from build123d import *

# Parameters (mm, degrees)
F0_R     = 2.5
F3_DEPTH = 24
F1_R     = 11
F4_DEPTH = 2
F5_DEPTH = 47
F7_D     = 4


with BuildPart() as f3:
    # F0 (on Front) → F3 (new body)
    with BuildSketch(Plane.XZ):
        Circle(F0_R)
    extrude(amount=F3_DEPTH)

    # F1 (on Front) → F4 (join)
    with BuildSketch(Plane.XZ):
        Circle(F1_R)
    extrude(amount=F4_DEPTH)

    # F2 (on Front) → F5 (join)
    with BuildSketch(Plane.XZ):
        Polygon((21, 16.5), (16.5, 21), (-16.5, 21), (-21, 16.5), (-21, -16.5), (-16.5, -21), (16.5, -21), (21, -16.5), align=None)
    extrude(amount=-F5_DEPTH)

    # F7 (through all)
    with Locations(Plane.XZ):
        with Locations((-15.5, 15.5), (15.5, 15.5), (15.5, -15.5), (-15.5, -15.5)):
            Hole(F7_D / 2)


solid = f3.part
For this review, take the finished solid that the model builds, in its own axes (mm). A direction names the side the tool comes from. Round coordinates to 2 decimals unless told otherwise and drop trailing zeros. Write each loop counter-clockwise with the first axis right and the second up, starting at its lowest first coordinate (ties: lowest second). Pieces come first, ordered by that corner, then holes. Notation, with made-up numbers: (38, -32) -> (43, -32) arc R28 ccw to (43, 4) -> close; hole circle Ø9 at (73, 39). An arc over 180 degrees is marked (long way). Put each result on its own line as item: value.
Q1. To check wall thickness, follow L1, parallel to Z at x = 15.5, y = 15; L2, parallel to Z at x = 15, y = 32. State the ranges of each line that lie inside material, in increasing order. Write a range as [from, to].
Determined:
L1: z = [-21, -17.5], [-13.5, 13.5], [17.5, 21]
L2: z = [-21, -17.44], [-13.56, 13.56], [17.44, 21]
Q2. Consider section D-D on x = 0. State the section outline as (y, z) points, and give its area (3 significant figures).
Determined:
outline: (-24, -2.5) -> (-2, -2.5) -> (-2, -11) -> (0, -11) -> (0, -21) -> (47, -21) -> (47, 21) -> (0, 21) -> (0, 11) -> (-2, 11) -> (-2, 2.5) -> (-24, 2.5) -> close
area: 2,130 mm^2
Q3. Consider section B-B on y = 42. State the section outline as (x, z) points.
Determined:
outline: (-21, -16.5) -> (-16.5, -21) -> (16.5, -21) -> (21, -16.5) -> (21, 16.5) -> (16.5, 21) -> (-16.5, 21) -> (-21, 16.5) -> close; hole circle Ø4 at (-15.5, -15.5); hole circle Ø4 at (-15.5, 15.5); hole circle Ø4 at (15.5, -15.5); hole circle Ø4 at (15.5, 15.5)
Q4. Machinability: for faces 1 (the flat face through (9, 0, -9)), 2 (the flat face through (0, 23, -21)), which of the approach directions +Z, -Z, +X, -X, +Y, -Y give a long, thin tool a straight path to every point of the face, cutting with its end or side? Answer none if there is none.
Determined:
face 1: -Y
face 2: -Z, +X, -X, +Y, -Y
Q5. Consider section C-C on z = 15.5. State the section outline as (x, y) points.
Determined:
outline: (-21, 0) -> (-17.5, 0) -> (-17.5, 47) -> (-21, 47) -> close; (-13.5, 0) -> (13.5, 0) -> (13.5, 47) -> (-13.5, 47) -> close; (17.5, 0) -> (21, 0) -> (21, 47) -> (17.5, 47) -> close
Q6. The part is to be moulded in two halves that separate along X. For faces 3 (the flat face through (21, 23, 0)), 4 (the cylindrical face through (-15.24, 23.829, 17.483)), 5 (the flat face through (-18.7, 23.2, 18.8)), say which applies: released by +X, released by -X, zero draft, split by the parting line, or undercut.
Determined:
face 3: released by +X
face 4: undercut
face 5: released by -X
Q7. Consider section A-A on x = 15.5. State the section outline as (y, z) points, and give its area (3 significant figures).
Determined:
outline: (0, -21) -> (47, -21) -> (47, -17.5) -> (0, -17.5) -> close; (0, -13.5) -> (47, -13.5) -> (47, 13.5) -> (0, 13.5) -> close; (0, 17.5) -> (47, 17.5) -> (47, 21) -> (0, 21) -> close
area: 1,600 mm^2
Q8. Clearance check with flat-ended pins moving along their axes: pin 1 Ø10 at (x, z) = (-5.5, 16) entering from -Y; pin 2 Ø3.5 at (x, z) = (15.5, -15.5) entering from +Y; pin 3 Ø10 at (x, y) = (1.5, -13) entering from +Z. State where each tip first meets the part, or that it passes through.
Determined:
pin 1: stops at y = 0
pin 2: passes through
pin 3: stops at z = 2.5
